Geometry: see drawing. Coordinates: mm, zero at the bounding-box minimum. Round coordinates to 2 decimals unless told otherwise and drop trailing zeros. Order: outer loops, then holes, each group sorted by start corner. A loop starts at its lowest first (then second) coordinate and runs counter-clockwise, first axis right, second up. Notation, with made-up numbers: (70.5, 79) -> (124.5, 79) arc R24 ccw to (124.5, 118) -> close; hole circle Ø2 at (27.25, 29). An arc over 180 degrees is marked (long way). Use a Markdown table: item, result.
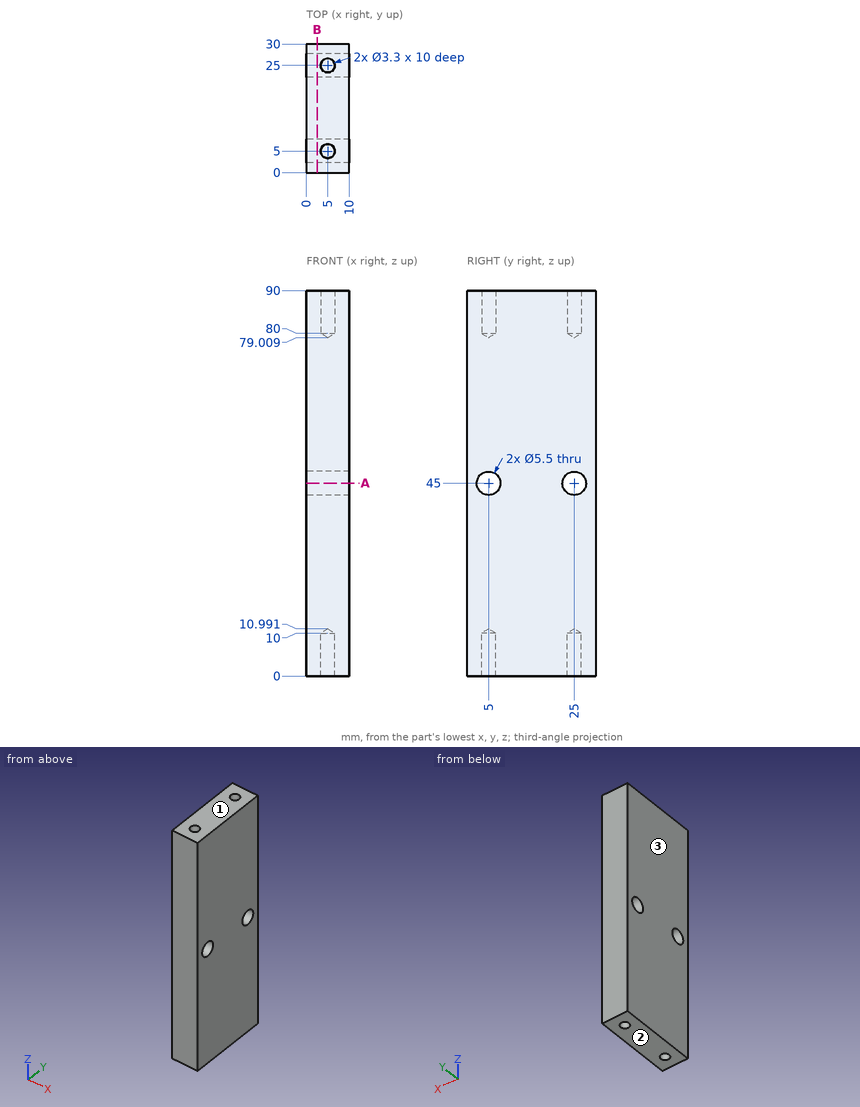
1) Contact query for flat-ended pins moving along their axis: P1, Ø2.5, axis at x = 5, y = 25, coming from the -Z side; P2, Ø2, axis at x = 5, y = 25, coming from the +Z side; P3, Ø2, axis at x = 5, y = 5, coming from the -Z side. Output: stop coordinate, or through.
Answer key:
| item | result |
|---|---|
| P1 | stops at z = 10.24 |
| P2 | stops at z = 79.61 |
| P3 | stops at z = 10.39 |
2) Ray query, probe 1 along Y at (x, z) = (5, 82.5); probe 2 along Y at (x, z) = (7.25, 45); probe 3 along X at (y, z) = (5.25, 9.5). Return the intervals inside material, ascending.
Answer key:
| item | result |
|---|---|
| probe 1 | y = 0 to 3.35, 6.65 to 23.35, 26.65 to 30 |
| probe 2 | y = 0 to 2.25, 7.75 to 22.25, 27.75 to 30 |
| probe 3 | x = 0 to 3.37, 6.63 to 10 |
3) Cut plane B-B on x = 2.5. Return loops of the section in (y, z), and give its area (3 significant figures).
Answer key:
| item | result |
|---|---|
| outline | (0, 0) -> (30, 0) -> (30, 90) -> (0, 90) -> close; hole circle Ø5.5 at (5, 45); hole circle Ø5.5 at (25, 45) |
| area | 2,650 mm^2 |
4) Draft query along Z for the marked faces 1, 2 and 3. Return one class per face: released by +Z, released by -Z, zero draft, split by the parting line, or undercut.
Answer key:
| item | result |
|---|---|
| face 1 | released by +Z |
| face 2 | released by -Z |
| face 3 | zero draft |
5) Cut plane A-A on z = 45. Return loops of the section in (x, y).
Answer key:
| item | result |
|---|---|
| outline | (0, 0) -> (10, 0) -> (10, 2.25) -> (0, 2.25) -> close; (0, 7.75) -> (10, 7.75) -> (10, 22.25) -> (0, 22.25) -> close; (0, 27.75) -> (10, 27.75) -> (10, 30) -> (0, 30) -> close |
